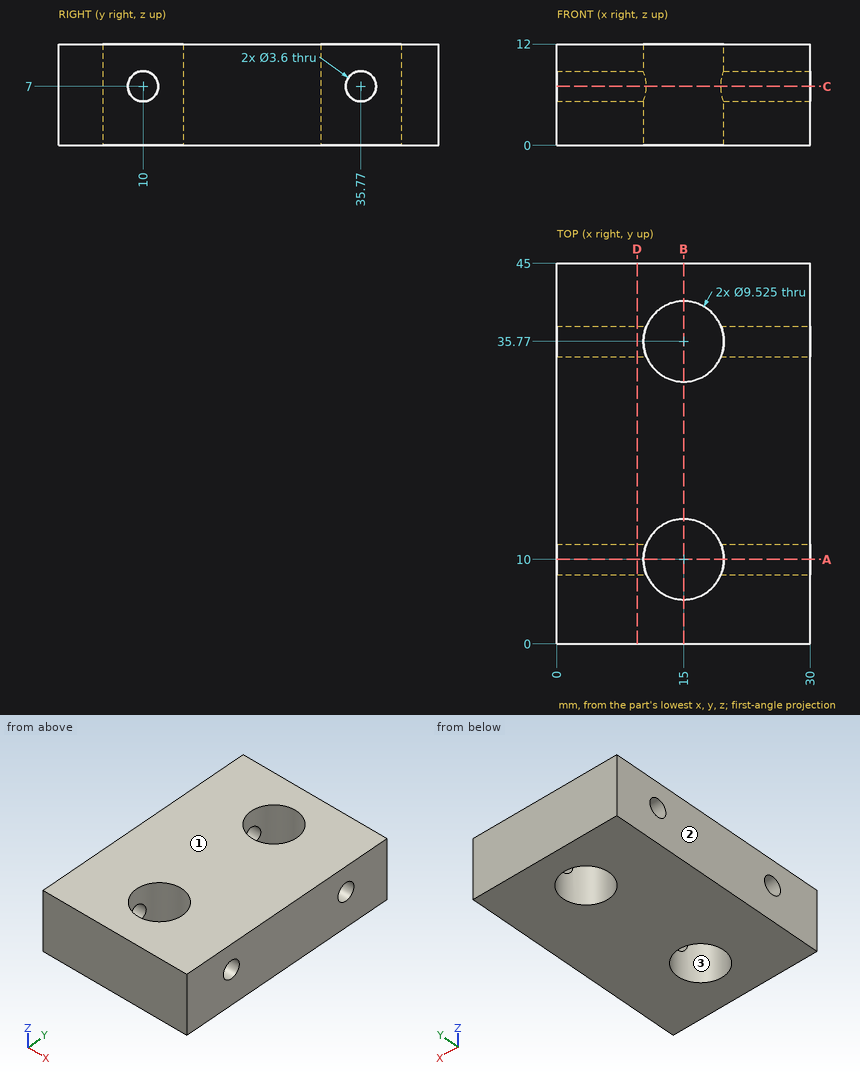
Geometry: see drawing. Coordinates: mm, zero at the bounding-box minimum. Coordinates: 2 decimals unless noted, no trailing zeros. Loops run counter-clockwise (first coordinate to the right, second up) from the corner with the lowest first, then second, coordinate; pieces in that order, holes last. Notation, with made-up numbers: M 10,21.25 L 41,21.25 A15 cw 41,38.25 Z; hole C -19,2.25 d8. An arc over 180 degrees is marked long. Put each result on its own line as item: value. Start each with the question number.
1) Cut plane A-A on y = 10. Return the cut outline in (x, z).
2) Cut plane B-B on x = 15. Return the cut outline in (y, z).
3) Ray query, L1, parallel to Y at x = 2.75, z = 7; L2, parallel to Z at x = 2.25, y = 35.77; L3, parallel to X at y = 37.5, z = 8.5. Return the intervals inside material, ascending. Write a range as from..to.
4) Pull-direction query (X, two-part tool) for the marked faces 1, 2 and 3; classes: pulls with the +X half, pulls with the -X half, needs draft (parallel to the pull), parting line crosses it, or undercut.
5) Cut plane D-D on x = 9.5. Return the cut outline in (y, z), then the cut area to 3 significant figures.
6) Cut plane C-C on z = 7. Return the cut outline in (x, y) (1 decimal).
The answers:
1. outline: M 0,0 L 10.24,0 L 10.24,5.2 L 0,5.2 Z; M 0,8.8 L 10.24,8.8 L 10.24,12 L 0,12 Z; M 19.76,0 L 30,0 L 30,5.2 L 19.76,5.2 Z; M 19.76,8.8 L 30,8.8 L 30,12 L 19.76,12 Z
2. outline: M 0,0 L 5.24,0 L 5.24,12 L 0,12 Z; M 14.76,0 L 31.01,0 L 31.01,12 L 14.76,12 Z; M 40.53,0 L 45,0 L 45,12 L 40.53,12 Z
3. L1: y = 0..8.2, 11.8..33.97, 37.57..45
3. L2: z = 0..5.2, 8.8..12
3. L3: x = 0..10.56, 19.44..30
4. face 1: needs draft
4. face 2: pulls with the -X half
4. face 3: undercut
5. outline: M 0,0 L 45,0 L 45,12 L 0,12 Z; hole C 10,7 d3.6; hole C 35.77,7 d3.6
5. area: 520 mm²
6. outline: M 0,0 L 30,0 L 30,8.2 L 19.4,8.2 A4.8 cw 10.6,8.2 L 0,8.2 Z; M 0,11.8 L 10.6,11.8 A4.8 cw 19.4,11.8 L 30,11.8 L 30,34 L 19.4,34 A4.8 cw 10.6,34 L 0,34 Z; M 0,37.6 L 10.6,37.6 A4.8 cw 19.4,37.6 L 30,37.6 L 30,45 L 0,45 Z
